```python
from build123d import *

# Parameters (mm, degrees)
SKETCH_1_W          = 16
SKETCH_1_H          = 18
EXTRUDE_1_DEPTH     = 4
SKETCH_2_R          = 1.65
CUT_EXTRUDE_1_DEPTH = 4
SKETCH_3_W          = 16
SKETCH_3_H          = 6
EXTRUDE_2_DEPTH     = 8
SKETCH_4_R          = 1.45
CUT_EXTRUDE_2_DEPTH = 27.907248094
CHAMFER_1_SIZE      = 3
CHAMFER_2_SIZE      = 3
CHAMFER_3_SIZE      = 3
SKETCH_6_R          = 3
CUT_EXTRUDE_3_DEPTH = 26.377155081
SKETCH_7_R          = 6.25
CUT_EXTRUDE_4_DEPTH = 2.8
CHAMFER_4_SIZE      = 1.5


with BuildPart() as part:
    # 草图1 → 凸台-拉伸1 (new body)
    with BuildSketch(Plane(origin=(0, 0, 0), x_dir=(1, 0, 0), z_dir=(0, 1, 0))):
        with Locations((8, 9)):
            Rectangle(SKETCH_1_W, SKETCH_1_H)
    extrude(amount=EXTRUDE_1_DEPTH)

    # 草图2 → 切除-拉伸1 (cut)
    with BuildSketch(Plane(origin=(0, 4, 0), x_dir=(1, 0, 0), z_dir=(0, 1, 0))):
        with Locations(Location((8, 10, 0), (0, 0, 270))):
            Circle(SKETCH_2_R)
    extrude(amount=-CUT_EXTRUDE_1_DEPTH, mode=Mode.SUBTRACT)

    # 草图3 → 凸台-拉伸2 (add)
    with BuildSketch(Plane(origin=(0, 4, 0), x_dir=(1, 0, 0), z_dir=(0, 1, 0))):
        with Locations((8, 3)):
            Rectangle(SKETCH_3_W, SKETCH_3_H)
    extrude(amount=EXTRUDE_2_DEPTH)

    # 草图4 → 切除-拉伸2 (cut, through all)
    with BuildSketch(Plane(origin=(0, 12, 0), x_dir=(1, 0, 0), z_dir=(0, 1, 0))):
        with Locations(Location((8, 2.4, 0), (0, 0, 270))):
            Circle(SKETCH_4_R)
    extrude(amount=-CUT_EXTRUDE_2_DEPTH, mode=Mode.SUBTRACT)

    # 倒角1
    chamfer_1_edges = [part.edges().sort_by_distance(p)[0] for p in [
        (0, 2, -18),
        (16, 2, -18),
    ]]
    chamfer(chamfer_1_edges, length=CHAMFER_1_SIZE)

    # 倒角2
    # the kernel refuses this chamfer: 3 mm, written as the material it adds along each edge
    with BuildSketch(Plane(origin=(16, 4, -6), x_dir=(0, -0.02749587661058635, -0.9996219169112968), z_dir=(-1, 0, 0))) as chamfer_2_piece_1_section:
        Polygon((CHAMFER_2_SIZE * 0.999621916911, -CHAMFER_2_SIZE * 0.0274958766106), (-CHAMFER_2_SIZE * 0.0274958766106, -CHAMFER_2_SIZE * 0.999621916911), (0, 0), align=None)
    chamfer_2_piece_1 = extrude(amount=16, mode=Mode.PRIVATE)
    chamfer_2_piece_1 = chamfer_2_piece_1 - Plane(origin=(8, 4.994786575, -10), x_dir=(0, 0, 1), z_dir=(0, 1, 0)) * Cylinder(1.65, 44, mode=Mode.PRIVATE)
    add(chamfer_2_piece_1)

    # 倒角3
    chamfer_3_edges = [part.edges().sort_by_distance(p)[0] for p in [
        (0, 12, -3),
        (16, 12, -3),
    ]]
    chamfer(chamfer_3_edges, length=CHAMFER_3_SIZE)

    # 草图6 → 切除-拉伸3 (cut, through all)
    with BuildSketch(Plane(origin=(0, 4, 0), x_dir=(1, 0, 0), z_dir=(0, 1, 0))):
        with Locations((8, 10)):
            Circle(SKETCH_6_R)
    extrude(amount=CUT_EXTRUDE_3_DEPTH, mode=Mode.SUBTRACT)

    # 草图7 → 切除-拉伸4 (cut)
    with BuildSketch(Plane(origin=(0, 0, 0), x_dir=(-1, 0, 0), z_dir=(0, -1, 0))):
        with Locations((-8, -4.5)):
            Circle(SKETCH_7_R)
    extrude(amount=-CUT_EXTRUDE_4_DEPTH, mode=Mode.SUBTRACT)

    # 倒角4
    # the kernel refuses this chamfer: 1.5 mm, written as the material it takes off along each edge
    with BuildSketch(Plane(origin=(16.194862375, 2.8, 0), x_dir=(0, 0.9996219169112969, 0.027495876610586382), z_dir=(-1, 0, 0))) as chamfer_4_piece_1_section:
        Polygon((CHAMFER_4_SIZE * 0.999621916911, CHAMFER_4_SIZE * 0.0274958766106), (-CHAMFER_4_SIZE * 0.0274958766106, CHAMFER_4_SIZE * 0.999621916911), (0, 0), align=None)
    chamfer_4_piece_1 = extrude(amount=16.38972475, mode=Mode.PRIVATE)
    chamfer_4_piece_1 = chamfer_4_piece_1 & Plane(origin=(8, 3.325118299, 4.5), x_dir=(-1, 0, 0), z_dir=(0, -1, 0)) * Cylinder(6.25, 39, mode=Mode.PRIVATE)
    add(chamfer_4_piece_1, mode=Mode.SUBTRACT)


solid = part.part
```
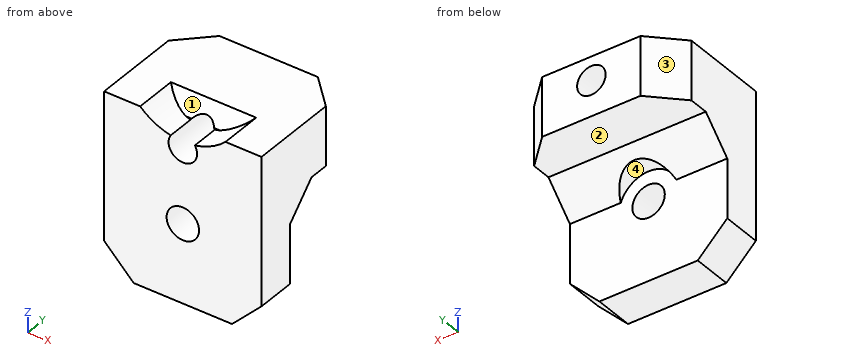
Check sheet for the modelled part. Datum: model origin and axes. Units: mm. Face numbers are marked on the shaded views. A direction names the side the tool comes from. Give positions to 0.01 mm unless a question says otherwise; leave off trailing zeros. Order: outer loops, then holes, each group sorted by start corner. A loop starts at its lowest first (then second) coordinate and runs counter-clockwise, first axis right, second up. Notation, with made-up numbers: (-9, -13) -> (7, -13) arc R12 ccw to (7, 10) -> close; hole circle Ø8 at (-5.75, 57). An arc over 180 degrees is marked (long way). Use CSV: the item, a comma, the result in double quotes. Start each with the question number.
1) Sectioned sample at C-C, the plane y = 6.5. Record the boundary of the cut face in (x, z).
2) Sectioned sample at A-A, the plane z = -10. Record the boundary of the cut face in (x, y), plus the area to 3 significant figures.
3) Sectioned sample at B-B, the plane x = 8. Record the boundary of the cut face in (y, z), plus the area to 3 significant figures.
4) Set-up check for the marked faces 1, 2, 3 and 4: record each of +Z, -Z, +X, -X, +Y, -Y from which the full face is reachable in a straight line by a thin tool's end or side.
5) Sectioned sample at D-D, the plane z = -2.4. Record the boundary of the cut face in (x, y).
6) Go/stop test with flat-tipped pins: P1, Ø4, axis at x = 14.5, z = -11.5, coming from the -Y side; P2, Ø1.5, axis at x = 13, z = -9, coming from the +Y side; P3, Ø4, axis at x = 10, y = 9.5, coming from the -Z side; P4, Ø5.5, axis at x = 8, y = 8.5, coming from the -Z side. Record where each tip stops, or that it passes through.
7) Material ranges on line 1 (X direction, y = 3, z = -2.4); line 2 (Z direction, x = 8, y = 3.05); line 3 (X direction, y = 2.75, z = -10), recorded low to high. Write a range as from..to.
Recorded:
1,outline,"(0, -6.5) -> (16, -6.5) -> (16, 0) -> (0, 0) -> close; hole circle Ø2.9 at (8, -2.4)"
2,outline,"(0, 0) -> (6.35, 0) -> (6.35, 4) -> (0, 4) -> close; (9.65, 0) -> (16, 0) -> (16, 4) -> (9.65, 4) -> close"
2,area,"50.8 mm2"
3,outline,"(0, -18) -> (4, -18) -> (4, -11.65) -> (0, -11.65) -> close; (0, -8.35) -> (4, -8.35) -> (4, -7) -> (6, -7) -> (7, -6) -> (12, -6) -> (12, -3.85) -> (0, -3.85) -> close; (3.35, -0.95) -> (12, -0.95) -> (12, 0) -> (4.3, 0) -> close"
3,area,"70.9 mm2"
4,face 1,"+Z, -Y"
4,face 2,"-Z, +X, -X, +Y"
4,face 3,"+Z, -Z, -X, +Y"
4,face 4,"-Z, +Y"
5,outline,"(0, 0) -> (6.55, 0) -> (6.55, 12) -> (3, 12) -> (0, 9) -> close; (9.45, 0) -> (16, 0) -> (16, 9) -> (13, 12) -> (9.45, 12) -> close"
6,P1,"y = 0"
6,P2,"y = 4.75"
6,P3,"z = -6"
6,P4,"z = -7.12"
7,line 1,"0..6.55, 9.45..16"
7,line 2,"-18..-11.65, -8.35..-3.85"
7,line 3,"0..6.35, 9.65..16"
